Model file for the job. Use its own axes, mm. Face numbers are marked on the shaded views. Give positions to 0.01 mm unless a question says otherwise; leave off trailing zeros. Write each loop counter-clockwise with the first axis right and the second up, starting at its lowest first coordinate (ties: lowest second). Pieces come first, ordered by that corner, then holes.
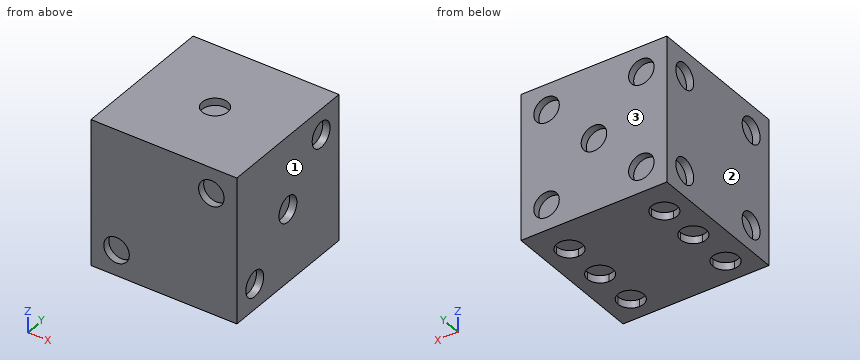
```python
from build123d import *

# Parameters (mm, degrees)
F0_W      = 127
F0_H      = 127
F1_DEPTH  = 127
F2_R      = 11.1125
F3_DEPTH  = 6.35
F4_R      = 11.1125
F5_DEPTH  = 6.35
F6_R      = 11.1125
F7_DEPTH  = 6.35
F9_R      = 11.1125
F10_DEPTH = 6.35
F12_DEPTH = 6.35
F8_R      = 11.1125
F13_DEPTH = 6.35


with BuildPart() as f1:
    # F0 (on Top) → F1 (new body)
    with BuildSketch(Plane.XY):
        with Locations((63.5, 63.5)):
            Rectangle(F0_W, F0_H)
    extrude(amount=F1_DEPTH)

    # F2 (on face) → F3 (cut)
    with BuildSketch(Plane.XY.offset(127)):
        with Locations((63.5, 63.5)):
            Circle(F2_R)
    extrude(amount=-F3_DEPTH, mode=Mode.SUBTRACT)

    # F4 (on face) → F5 (cut)
    with BuildSketch(Plane.XZ):
        with Locations((22.225, 22.225)):
            Circle(F4_R)
        with Locations((104.775, 104.775)):
            Circle(F4_R)
    extrude(amount=-F5_DEPTH, mode=Mode.SUBTRACT)

    # F6 (on face) → F7 (cut)
    with BuildSketch(Plane.YZ.offset(127)):
        with Locations((22.225, 22.225)):
            Circle(F6_R)
        with Locations((63.5, 63.5)):
            Circle(F6_R)
        with Locations((104.775, 104.775)):
            Circle(F6_R)
    extrude(amount=-F7_DEPTH, mode=Mode.SUBTRACT)

    # F9 (on face) → F10 (cut)
    with BuildSketch(Plane(origin=(0, 0, 0), x_dir=(0, -1, 0), z_dir=(-1, 0, 0))):
        with Locations((-104.775, 104.775)):
            Circle(F9_R)
        with Locations((-22.225, 104.775)):
            Circle(F9_R)
        with Locations((-104.775, 22.225)):
            Circle(F9_R)
        with Locations((-22.225, 22.225)):
            Circle(F9_R)
    extrude(amount=-F10_DEPTH, mode=Mode.SUBTRACT)

    # F11 (on face) → F12 (cut)
    with BuildSketch(Plane(origin=(0, 0, 0), x_dir=(1, 0, 0), z_dir=(0, 0, -1))):
        with BuildLine():
            ThreePointArc((33.3375, -22.225), (30.082724, -14.367276), (22.225, -11.1125))
            Line((22.225, -11.1125), (22.225, -33.3375))
            ThreePointArc((22.225, -33.3375), (30.082724, -30.082724), (33.3375, -22.225))
        make_face()
        with BuildLine():
            ThreePointArc((33.3375, -98.425), (30.082724, -90.567276), (22.225, -87.3125))
            Line((22.225, -87.3125), (22.225, -109.5375))
            ThreePointArc((22.225, -109.5375), (30.082724, -106.282724), (33.3375, -98.425))
        make_face()
        with BuildLine():
            Line((22.225, -109.5375), (22.225, -87.3125))
            ThreePointArc((22.225, -87.3125), (11.1125, -98.425), (22.225, -109.5375))
        make_face()
        with BuildLine():
            ThreePointArc((33.3375, -62.355265), (30.082724, -54.497541), (22.225, -51.242765))
            Line((22.225, -51.242765), (22.225, -73.467765))
            ThreePointArc((22.225, -73.467765), (30.082724, -70.212989), (33.3375, -62.355265))
        make_face()
        with BuildLine():
            Line((22.225, -73.467765), (22.225, -51.242765))
            ThreePointArc((22.225, -51.242765), (11.1125, -62.355265), (22.225, -73.467765))
        make_face()
        with BuildLine():
            Line((22.225, -33.3375), (22.225, -11.1125))
            ThreePointArc((22.225, -11.1125), (11.1125, -22.225), (22.225, -33.3375))
        make_face()
        with BuildLine():
            ThreePointArc((115.8875, -22.225), (112.632724, -14.367276), (104.775, -11.1125))
            Line((104.775, -11.1125), (104.775, -33.3375))
            ThreePointArc((104.775, -33.3375), (112.632724, -30.082724), (115.8875, -22.225))
        make_face()
        with BuildLine():
            ThreePointArc((115.8875, -98.425), (112.632724, -90.567276), (104.775, -87.3125))
            Line((104.775, -87.3125), (104.775, -109.5375))
            ThreePointArc((104.775, -109.5375), (112.632724, -106.282724), (115.8875, -98.425))
        make_face()
        with BuildLine():
            Line((104.775, -109.5375), (104.775, -87.3125))
            ThreePointArc((104.775, -87.3125), (93.6625, -98.425), (104.775, -109.5375))
        make_face()
        with BuildLine():
            ThreePointArc((115.8875, -60.325), (112.632724, -52.467276), (104.775, -49.2125))
            Line((104.775, -49.2125), (104.775, -71.4375))
            ThreePointArc((104.775, -71.4375), (112.632724, -68.182724), (115.8875, -60.325))
        make_face()
        with BuildLine():
            Line((104.775, -71.4375), (104.775, -49.2125))
            ThreePointArc((104.775, -49.2125), (93.6625, -60.325), (104.775, -71.4375))
        make_face()
        with BuildLine():
            Line((104.775, -33.3375), (104.775, -11.1125))
            ThreePointArc((104.775, -11.1125), (93.6625, -22.225), (104.775, -33.3375))
        make_face()
    extrude(amount=-F12_DEPTH, mode=Mode.SUBTRACT)

    # F8 (on face) → F13 (cut)
    with BuildSketch(Plane(origin=(0, 127, 0), x_dir=(-1, 0, 0), z_dir=(0, 1, 0))):
        with Locations((-63.5, 63.5)):
            Circle(F8_R)
        with Locations((-104.775, 104.775)):
            Circle(F8_R)
        with Locations((-22.225, 104.775)):
            Circle(F8_R)
        with Locations((-104.775, 22.225)):
            Circle(F8_R)
        with Locations((-22.225, 22.225)):
            Circle(F8_R)
    extrude(amount=-F13_DEPTH, mode=Mode.SUBTRACT)


solid = f1.part
```
1. Slice it at C-C, the plane y = 101. Write the cut outline in (x, z), and give its area (3 significant figures).
Calculated:
outline: (0, 0) - (11.41, 0) - (11.41, 6.35) - (33.04, 6.35) - (33.04, 0) - (93.96, 0) - (93.96, 6.35) - (115.59, 6.35) - (115.59, 0) - (127, 0) - (127, 94.32) - (120.65, 94.32) - (120.65, 115.23) - (127, 115.23) - (127, 127) - (0, 127) - (0, 115.23) - (6.35, 115.23) - (6.35, 94.32) - (0, 94.32) - (0, 32.68) - (6.35, 32.68) - (6.35, 11.77) - (0, 11.77) - close
area: 15,500 mm2
2. Slice it at A-A, the plane z = 63.5. Write the cut outline in (x, y).
Calculated:
outline: (0, 0) - (127, 0) - (127, 52.39) - (120.65, 52.39) - (120.65, 74.61) - (127, 74.61) - (127, 127) - (74.61, 127) - (74.61, 120.65) - (52.39, 120.65) - (52.39, 127) - (0, 127) - close
3. Probe probe 1 along Y at (x, z) = (63.5, 125.5); probe 2 along Z at (x, y) = (100, 89); probe 3 along Z at (x, y) = (55, 61). List the from-to ranges inside material, lowest first.
Calculated:
probe 1: y = 0 to 52.39, 74.61 to 127
probe 2: z = 6.35 to 127
probe 3: z = 0 to 120.65
4. Pull direction X, two halves, no side cores. Call the marked faces 1, 2 and 3: +X half, -X half, draft (parallel to the pull), parting line (faces both ways), or undercut.
Calculated:
face 1: +X half
face 2: -X half
face 3: draft
5. Slice it at D-D, the plane y = 57.5. Write the cut outline in (x, z), and give its area (3 significant figures).
Calculated:
outline: (0, 0) - (12.23, 0) - (12.23, 6.35) - (32.22, 6.35) - (32.22, 0) - (94.03, 0) - (94.03, 6.35) - (115.52, 6.35) - (115.52, 0) - (127, 0) - (127, 54.15) - (120.65, 54.15) - (120.65, 72.85) - (127, 72.85) - (127, 127) - (72.85, 127) - (72.85, 120.65) - (54.15, 120.65) - (54.15, 127) - (0, 127) - close
area: 15,600 mm2
6. Pin check, flat tips, straight feed: P1, Ø20, axis at x = 22.225, z = 104.775, coming from the +Y side; P2, Ø11, axis at x = 21, y = 101, coming from the -Z side; P3, Ø20, axis at y = 104.775, z = 104.775, coming from the -X side. Stop position of each tip, or through.
Calculated:
P1: stops at y = 120.65
P2: stops at z = 6.35
P3: stops at x = 6.35
